The listing builds one solid part. Answer for the finished solid, in the listing's coordinates (mm). Give positions to 0.01 mm unless a question says otherwise; leave off trailing zeros. Order: outer loops, then holes, each group sorted by start corner. A loop starts at its lowest first (then second) coordinate and runs counter-clockwise, first axis right, second up. Notation, with made-up numbers: (0, 34.25) - (12, 34.25) arc R23 cw to (12, 73.25) - close; hole circle Ø7 at (45.5, 32). An arc over 180 degrees is marked (long way). Answer as CSV lines item,"result". Start each with the question number.
1. Consider line 1 along Y through (x, z) = (98.5, 1.75); line 2 along X through (y, z) = (20.5, 3); line 3 along Y through (x, z) = (-122, 6). Determine where each line is inside the solid, lowest interval first. Write a range as [from, to].
2. Determine the mould class of faces 1 (the cylindrical face through (-40.838, 32.401, 5.916)), 2 (the flat face through (163.486, 26.4, 4.6)), 3 (the flat face through (13, 28, 12)) for opening direction X: +X half, -X half, draft (parallel to the pull), parting line (faces both ways), or undercut.
3. Section A-A on y = 11 is taken. Give the vertices of the cut face in (x, z), and give its area (3 significant figures).
4. Flat-ended cylindrical pins translate along their axes: pin 1 (5 mm diameter, centred on x = 69.49, y = 29.7, fed in from -Z); pin 2 (5.5 mm diameter, centred on x = 93.49, y = -25.7, fed in from -Z); pin 3 (2.5 mm diameter, centred on y = 27.3, z = 6, fed in from +X); pin 4 (1.5 mm diameter, centred on y = 27.5, z = 6.5, fed in from -X). Find the tip coordinate at first contact, or state that the pin passes through.
5. Section B-B on z = 9.5 is taken. Give the vertices of the cut face in (x, y), and give its area (3 significant figures).
from build123d import *

# Parameters (mm, degrees)
SKETCH1_W           = 296
SKETCH1_H           = 126
SKETCH1_R           = 16
SKETCH1_R_2         = 7
SKETCH1_R_3         = 1.5
SKETCH1_R_4         = 3
BOSS_EXTRUDE1_DEPTH = 12
CUT_EXTRUDE1_START  = 90.297917
SKETCH2_R           = 1.5
CUT_EXTRUDE1_DEPTH  = 20
CUT_EXTRUDE3_START  = 163.485661
SKETCH3_R           = 1.5
CUT_EXTRUDE3_DEPTH  = 20
CUT_EXTRUDE4_START  = -132.514339
SKETCH3_2_R         = 1.5
CUT_EXTRUDE4_DEPTH  = 20
SKETCH4_R           = 3
CUT_EXTRUDE5_DEPTH  = 3
CUT_EXTRUDE5_TAPER  = 45


with BuildPart() as part:
    # Sketch1 → Boss-Extrude1 (new body)
    with BuildSketch(Plane.XY):
        with Locations((15.485661099, 27.29791691)):
            Rectangle(SKETCH1_W, SKETCH1_H)
        with Locations((93.485661099, 8.29791691)):
            Circle(SKETCH1_R, mode=Mode.SUBTRACT)
        with Locations((-47.514338901, 30.29791691)):
            Circle(SKETCH1_R_2, mode=Mode.SUBTRACT)
        with Locations((69.485661099, 29.69791691)):
            Circle(SKETCH1_R_3, mode=Mode.SUBTRACT)
        with Locations((117.485661099, 29.69791691)):
            Circle(SKETCH1_R_3, mode=Mode.SUBTRACT)
        with Locations((93.485661099, -25.70208309)):
            Circle(SKETCH1_R_4, mode=Mode.SUBTRACT)
    extrude(amount=BOSS_EXTRUDE1_DEPTH)

    # Sketch2 → Cut-Extrude1 (cut)
    with BuildSketch(Plane(origin=(0, 0, 0), x_dir=(1, 0, 0), z_dir=(0, 1, 0)).offset(CUT_EXTRUDE1_START)):
        with Locations((15.485661099, -6)):
            Circle(SKETCH2_R)
    extrude(amount=-CUT_EXTRUDE1_DEPTH, mode=Mode.SUBTRACT)

    # Sketch3 → Cut-Extrude3 (cut)
    with BuildSketch(Plane(origin=(0, 0, 0), x_dir=(0, 0, -1), z_dir=(1, 0, 0)).offset(CUT_EXTRUDE3_START)):
        with Locations((-6, 27.29791691)):
            Circle(SKETCH3_R)
    extrude(amount=-CUT_EXTRUDE3_DEPTH, mode=Mode.SUBTRACT)

    # Sketch3<2> → Cut-Extrude4 (cut)
    with BuildSketch(Plane(origin=(0, 0, 0), x_dir=(0, 0, -1), z_dir=(1, 0, 0)).offset(CUT_EXTRUDE4_START)):
        with Locations((-6, 27.29791691)):
            Circle(SKETCH3_2_R)
    extrude(amount=CUT_EXTRUDE4_DEPTH, mode=Mode.SUBTRACT)

    # Sketch4 → Cut-Extrude5 (cut)
    with BuildSketch(Plane.XY):
        with Locations((117.485661099, 29.69791691)):
            Circle(SKETCH4_R)
        with Locations((69.485661099, 29.69791691)):
            Circle(SKETCH4_R)
    extrude(amount=CUT_EXTRUDE5_DEPTH, taper=CUT_EXTRUDE5_TAPER, mode=Mode.SUBTRACT)


solid = part.part
Checks:
1,line 1,"y = [-35.7, -6.9], [23.49, 90.3]"
1,line 2,"x = [-132.51, 83.14], [103.84, 163.49]"
1,line 3,"y = [-35.7, 25.8], [28.8, 90.3]"
2,face 1,"undercut"
2,face 2,"+X half"
2,face 3,"draft"
3,outline,"(-132.51, 0) - (77.72, 0) - (77.72, 12) - (-132.51, 12) - close; (109.26, 0) - (163.49, 0) - (163.49, 12) - (109.26, 12) - close"
3,area,"3,170 mm²"
4,pin 1,"stops at z = 0.5"
4,pin 2,"passes through"
4,pin 3,"stops at x = 143.49"
4,pin 4,"stops at x = -112.51"
5,outline,"(-132.51, -35.7) - (163.49, -35.7) - (163.49, 90.3) - (-132.51, 90.3) - close; hole circle Ø14 at (-47.51, 30.3); hole circle Ø3 at (69.49, 29.7); hole circle Ø32 at (93.49, 8.3); hole circle Ø6 at (93.49, -25.7); hole circle Ø3 at (117.49, 29.7)"
5,area,"36,300 mm²"
